```python
from build123d import *

# Parameters (mm, degrees)
SKETCH1_W           = 355.6
SKETCH1_H           = 203.2
BOSS_EXTRUDE1_DEPTH = 6.35
SKETCH2_R           = 44.45
SKETCH2_R_2         = 3.96875
CUT_EXTRUDE1_DEPTH  = 76.2
SKETCH3_R           = 3.50012
CUT_EXTRUDE2_DEPTH  = 6.35
FILLET1_R           = 25.4
SKETCH5_R           = 3.175
CUT_EXTRUDE4_DEPTH  = 6.35


with BuildPart() as part:
    # Sketch1 → Boss-Extrude1 (new body)
    with BuildSketch(Plane.XY):
        with Locations((177.8, 101.6)):
            Rectangle(SKETCH1_W, SKETCH1_H)
    extrude(amount=BOSS_EXTRUDE1_DEPTH)

    # Sketch2 → Cut-Extrude1 (cut)
    with BuildSketch(Plane.XY.offset(6.35)):
        with Locations((76.2, 101.6)):
            Circle(SKETCH2_R)
        with Locations((143.66875, 101.6)):
            Circle(SKETCH2_R_2)
        with Locations((123.907610643, 53.892389357)):
            Circle(SKETCH2_R_2)
        with Locations((76.2, 34.13125)):
            Circle(SKETCH2_R_2)
        with Locations((28.492389357, 53.892389357)):
            Circle(SKETCH2_R_2)
        with Locations((8.73125, 101.6)):
            Circle(SKETCH2_R_2)
        with Locations((28.492389357, 149.307610643)):
            Circle(SKETCH2_R_2)
        with Locations((76.2, 169.06875)):
            Circle(SKETCH2_R_2)
        with Locations((123.907610643, 149.307610643)):
            Circle(SKETCH2_R_2)
    extrude(amount=-CUT_EXTRUDE1_DEPTH, mode=Mode.SUBTRACT)

    # Sketch3 → Cut-Extrude2 (cut)
    with BuildSketch(Plane.XY.offset(6.35)):
        with Locations((38.69944, 170.09999)):
            Circle(SKETCH3_R)
        with Locations((113.70056, 170.09999)):
            Circle(SKETCH3_R)
        with Locations((113.70056, 33.10001)):
            Circle(SKETCH3_R)
        with Locations((38.69944, 33.10001)):
            Circle(SKETCH3_R)
    extrude(amount=-CUT_EXTRUDE2_DEPTH, mode=Mode.SUBTRACT)

    # Fillet1
    fillet1_edges = [part.edges().sort_by_distance(p)[0] for p in [
        (0, 203.2, 3.175),
        (355.6, 203.2, 3.175),
        (355.6, 0, 3.175),
        (0, 0, 3.175),
    ]]
    fillet(fillet1_edges, radius=FILLET1_R)

    # Sketch5 → Cut-Extrude4 (cut)
    with BuildSketch(Plane(origin=(0, 0, 0), x_dir=(-1, 0, 0), z_dir=(0, 0, -1))):
        with Locations((-342.9, 114.3)):
            Circle(SKETCH5_R)
        with Locations((-190.5, 114.3)):
            Circle(SKETCH5_R)
        with Locations((-190.5, 38.1)):
            Circle(SKETCH5_R)
        with Locations((-342.9, 38.1)):
            Circle(SKETCH5_R)
    extrude(amount=-CUT_EXTRUDE4_DEPTH, mode=Mode.SUBTRACT)


solid = part.part
```
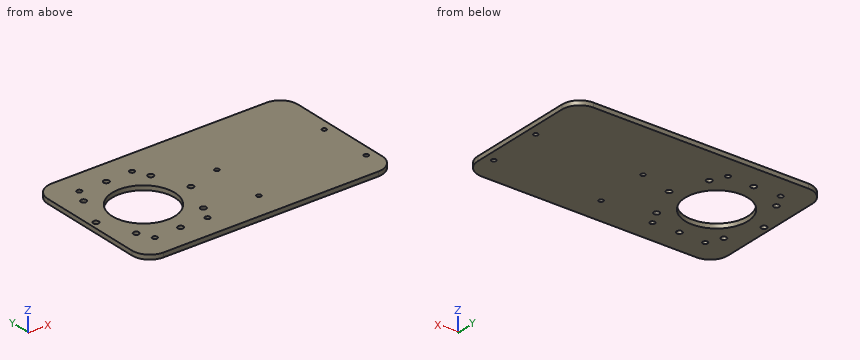
Build history of the part. All positions in model axes, mm. Give positions to 0.01 mm unless a question says otherwise; leave off trailing zeros. Loops run counter-clockwise (first coordinate to the right, second up) from the corner with the lowest first, then second, coordinate; pieces in that order, holes last.
Item 1: Drill centre lines: line 1 (Y direction, x = 76.2, z = 2.25); line 2 (X direction, y = 33.5, z = 3.25); line 3 (Y direction, x = 342.9, z = 3) (3 decimals). Where is each one in solid material? Low to high.
Answers follow:
line 1: y = 0 to 30.16, 38.1 to 57.15, 146.05 to 165.1, 173.04 to 203.2
line 2: x = 0 to 35.22, 42.18 to 72.28, 80.12 to 110.22, 117.18 to 355.6
line 3: y = 3.403 to 34.925, 41.275 to 111.125, 117.475 to 199.797
Item 2: Slice it at D-D, the plane z = 1. Give the number of separate pieces and of enclosed holes in the cut face, and give its area (3 significant figures).
Answers follow:
separate pieces: 1
enclosed holes: 17
area: 64,800 mm2
Item 3: Slice it at A-A, the plane x = 76.2. List the corners of the cut face in (y, z), and give its area (3 significant figures).
Answers follow:
outline: (0, 0) - (30.16, 0) - (30.16, 6.35) - (0, 6.35) - close; (38.1, 0) - (57.15, 0) - (57.15, 6.35) - (38.1, 6.35) - close; (146.05, 0) - (165.1, 0) - (165.1, 6.35) - (146.05, 6.35) - close; (173.04, 0) - (203.2, 0) - (203.2, 6.35) - (173.04, 6.35) - close
area: 625 mm2
Item 4: Slice it at C-C, the plane y = 124.5. List the corners of the cut face in (x, z), and give its area (3 significant figures).
Answers follow:
outline: (0, 0) - (38.1, 0) - (38.1, 6.35) - (0, 6.35) - close; (114.3, 0) - (355.6, 0) - (355.6, 6.35) - (114.3, 6.35) - close
area: 1,770 mm2
Item 5: Slice it at B-B, the plane y = 101.6. List the corners of the cut face in (x, z).
Answers follow:
outline: (0, 0) - (4.76, 0) - (4.76, 6.35) - (0, 6.35) - close; (12.7, 0) - (31.75, 0) - (31.75, 6.35) - (12.7, 6.35) - close; (120.65, 0) - (139.7, 0) - (139.7, 6.35) - (120.65, 6.35) - close; (147.64, 0) - (355.6, 0) - (355.6, 6.35) - (147.64, 6.35) - close
